Geometry: final body of the model. Coordinates: model frame, mm. Face numbers are marked on the shaded views. A direction names the side the tool comes from. Give positions to 0.01 mm unless a question says otherwise; leave off trailing zeros. Loops run counter-clockwise (first coordinate to the right, second up) from the corner with the lowest first, then second, coordinate; pieces in that order, holes last. Notation, with made-up numbers: (75, 67) -> (99, 67) arc R17 cw to (99, 74) -> close; hole circle Ø9 at (37, 81). An arc over 180 degrees is marked (long way). One line per item, written item: value. Start each with the question number.
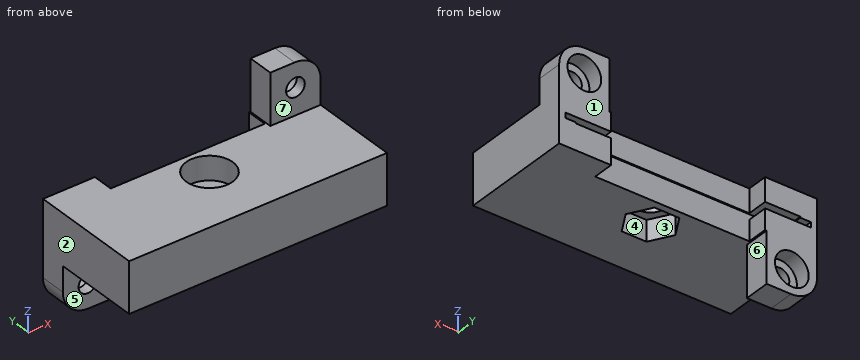
from build123d import *

# Parameters (mm, degrees)
BOSS_EXTRUDE1_DEPTH            = 4.85
SKETCH2_W                      = 43.3
SKETCH2_H                      = 0.2
CUT_EXTRUDE1_DEPTH             = 21
BOSS_EXTRUDE2_DEPTH            = 5
CBORE_FOR_M3_SHCS1_D           = 3.6
CBORE_FOR_M3_SHCS1_CBORE_D     = 6.5
CBORE_FOR_M3_SHCS1_CBORE_DEPTH = 3
CUT_EXTRUDE2_DEPTH             = 4
CUT_EXTRUDE3_REACH             = 59.668
SKETCH9_R                      = 4.5
SKETCH10_W                     = 8.8
SKETCH10_H                     = 1
CUT_EXTRUDE4_DEPTH             = 4
SKETCH11_R                     = 2.7
CUT_EXTRUDE5_DEPTH             = 0.95


with BuildPart() as part:
    # Sketch1 → Boss-Extrude1 (new, symmetric)
    with BuildSketch(Plane.XY):
        Polygon((0, 0), (0, 21.8), (10, 21.8), (10, 17.8), (39.7, 17.8), (39.7, 21.8), (49.7, 21.8), (49.7, 0), align=None)
    extrude(amount=BOSS_EXTRUDE1_DEPTH, both=True)

    # Sketch2 → Cut-Extrude1 (cut)
    with BuildSketch(Plane(origin=(0, 21.8, 0), x_dir=(1, 0, 0), z_dir=(0, 1, 0))):
        with Locations((24.85, -0.2)):
            Rectangle(SKETCH2_W, SKETCH2_H)
    extrude(amount=-CUT_EXTRUDE1_DEPTH, mode=Mode.SUBTRACT)

    # Sketch3 → Boss-Extrude2 (add)
    with BuildSketch(Plane(origin=(0, 21.8, 0), x_dir=(1, 0, 0), z_dir=(0, 1, 0))):
        with BuildLine():
            Line((0, 9.65), (0, 4.85))
            Line((0, 4.85), (9.7, 4.85))
            Line((9.7, 4.85), (9.7, 14.65))
            Line((9.7, 14.65), (5, 14.65))
            ThreePointArc((5, 14.65), (1.464466094, 13.185533906), (0, 9.65))
        make_face()
        with BuildLine():
            Line((49.7, -4.85), (40, -4.85))
            Line((40, -4.85), (40, -14.65))
            Line((40, -14.65), (44.7, -14.65))
            ThreePointArc((44.7, -14.65), (48.235533906, -13.185533906), (49.7, -9.65))
            Line((49.7, -9.65), (49.7, -4.85))
        make_face()
    extrude(amount=-BOSS_EXTRUDE2_DEPTH)

    # CBORE for M3 SHCS1 (through all)
    with Locations(Plane(origin=(0, 21.8, 0), x_dir=(1, 0, 0), z_dir=(0, 1, 0))):
        with Locations((44.85, -10), (4.85, 10)):
            CounterBoreHole(CBORE_FOR_M3_SHCS1_D / 2, CBORE_FOR_M3_SHCS1_CBORE_D / 2, CBORE_FOR_M3_SHCS1_CBORE_DEPTH)

    # Sketch7 → Cut-Extrude2 (cut)
    with BuildSketch(Plane(origin=(0, 0, -4.85), x_dir=(-1, 0, 0), z_dir=(0, 0, -1))):
        Polygon((-29.642007234, 12.3), (-27.246003617, 8.15), (-22.453996383, 8.15), (-20.057992766, 12.3), (-22.453996383, 16.45), (-27.246003617, 16.45), align=None)
    extrude(amount=-CUT_EXTRUDE2_DEPTH, mode=Mode.SUBTRACT)

    # Sketch9 → Cut-Extrude3 (cut, up to next)
    with BuildSketch(Plane.XY.offset(4.85), mode=Mode.PRIVATE) as cut_extrude3_sk1:
        with Locations((24.85, 12.3)):
            Circle(SKETCH9_R)
    cut_extrude3_tool1 = extrude(cut_extrude3_sk1.sketch, amount=-CUT_EXTRUDE3_REACH, mode=Mode.PRIVATE) & part.part
    add(cut_extrude3_tool1.solids().sort_by_distance((24.85, 12.3, 4.85))[0], mode=Mode.SUBTRACT)

    # Sketch10 → Cut-Extrude4 (cut)
    with BuildSketch(Plane(origin=(0, 21.8, 0), x_dir=(1, 0, 0), z_dir=(0, 1, 0))):
        with Locations((5.6, 0.4)):
            Rectangle(SKETCH10_W, SKETCH10_H)
        with Locations((44.1, -0.8)):
            Rectangle(SKETCH10_W, SKETCH10_H)
    extrude(amount=-CUT_EXTRUDE4_DEPTH, mode=Mode.SUBTRACT)

    # Sketch11 → Cut-Extrude5 (cut)
    with BuildSketch(Plane.XY.offset(0.1)):
        with Locations((24.85, 12.3)):
            Circle(SKETCH11_R)
    extrude(amount=-CUT_EXTRUDE5_DEPTH, mode=Mode.SUBTRACT)


solid = part.part
Item 1: Section C-C, the plane x = 24.85. Output: boundary loops of the cut face in (y, z).
Item 2: Ray query, line 1 along Z through (x, y) = (44.85, 20.8); line 2 along Z through (x, y) = (44.85, 17.3); line 3 along Y through (x, z) = (24.85, 3.85). Return the intervals inside material, ascending. Write a range as [from, to].
Item 3: Section D-D, the plane z = 3.25. Output: boundary loops of the cut face in (x, y), then the cut area to 3 significant figures.
Item 4: Access query for the marked faces 5, 6 and 7. Directions: +Z, -Z, +X, -X, +Y, -Y. A direction counts if a zero-diameter tool reaches every point of the face in a straight line with its end or side. Return the directions, or none.
Item 5: Pin query (flat end, axial travel): pin 1 (4 mm diameter, centred on x = 22, y = 17.5, fed in from +Z); pin 2 (2.5 mm diameter, centred on x = 12.5, z = -3.5, fed in from +Y); pin 3 (3 mm diameter, centred on x = 43.5, z = 9.5, fed in from +Y); pin 4 (3 mm diameter, centred on x = 17.5, z = 8, fed in from -Y). Return the tip coordinate at first contact, or that it passes through.
Item 6: Section A-A, the plane z = -3. Output: boundary loops of the cut face in (x, y).
Item 7: Mould query, pull axis Y, two halves, no side actions, for the marked faces 1, 2, 3 and 4. Classes: pulls with the +Y half, pulls with the -Y half, needs draft (parallel to the pull), parting line crosses it, or undercut.
Item 8: Section B-B, the plane y = 4. Output: boundary loops of the cut face in (x, z), then the cut area to 3 significant figures.
Geometry check:
1. outline: (0, -4.85) -> (8.15, -4.85) -> (8.15, -0.85) -> (9.6, -0.85) -> (9.6, 0.1) -> (0.8, 0.1) -> (0.8, 0.3) -> (7.8, 0.3) -> (7.8, 4.85) -> (0, 4.85) -> close; (15, -0.85) -> (16.45, -0.85) -> (16.45, -4.85) -> (17.8, -4.85) -> (17.8, 0.1) -> (15, 0.1) -> close; (16.8, 0.3) -> (17.8, 0.3) -> (17.8, 4.85) -> (16.8, 4.85) -> close
2. line 1: z = [-4.85, 0.1], [1.3, 6.75], [13.25, 14.65]
2. line 2: z = [-4.85, 0.1], [0.3, 8.2], [11.8, 14.65]
2. line 3: y = [0, 7.8], [16.8, 17.8]
3. outline: (0, 0) -> (49.7, 0) -> (49.7, 21.8) -> (39.7, 21.8) -> (39.7, 17.8) -> (10, 17.8) -> (10, 21.8) -> (0, 21.8) -> close; hole circle Ø9 at (24.85, 12.3)
3. area: 901 mm2
4. face 5: -Z, +X, -X, -Y
4. face 6: -Z, +X, +Y, -Y
4. face 7: +Z, +X, -X, -Y
5. pin 1: stops at z = 4.85
5. pin 2: stops at y = 17.8
5. pin 3: stops at y = 18.8
5. pin 4: passes through
6. outline: (0, 0) -> (49.7, 0) -> (49.7, 21.8) -> (39.7, 21.8) -> (39.7, 17.8) -> (10, 17.8) -> (10, 21.8) -> (0, 21.8) -> close; hole (20.06, 12.3) -> (22.45, 8.15) -> (27.25, 8.15) -> (29.64, 12.3) -> (27.25, 16.45) -> (22.45, 16.45) -> close
7. face 1: pulls with the +Y half
7. face 2: needs draft
7. face 3: undercut
7. face 4: undercut
8. outline: (0, -4.85) -> (49.7, -4.85) -> (49.7, 4.85) -> (0, 4.85) -> close; hole (3.2, 0.1) -> (46.5, 0.1) -> (46.5, 0.3) -> (3.2, 0.3) -> close
8. area: 473 mm2
